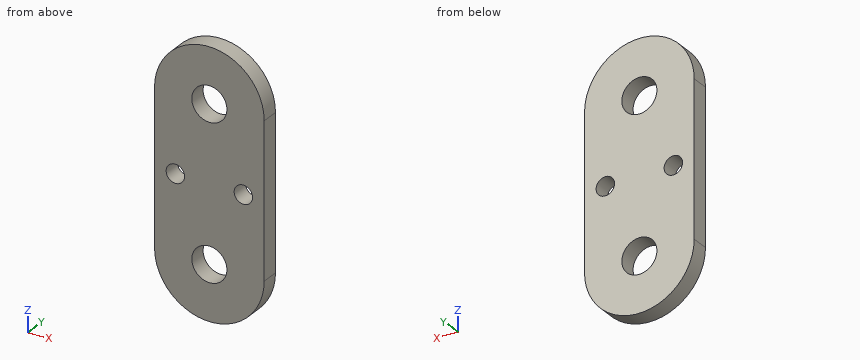
```python
from build123d import *

# Parameters (mm, degrees)
SKETCH1_R           = 12.5
SKETCH1_R_2         = 4
SKETCH1_R_3         = 2.1
BOSS_EXTRUDE1_DEPTH = 4


with BuildPart() as part:
    # Sketch1 → Boss-Extrude1 (new body)
    with BuildSketch(Plane(origin=(0, 0, 0), x_dir=(1, 0, 0), z_dir=(0, 1, 0))):
        with Locations((0, 17.5)):
            Circle(SKETCH1_R)
        with Locations((0, 17.5)):
            Circle(SKETCH1_R_2, mode=Mode.SUBTRACT)
        with BuildLine():
            ThreePointArc((-12.5, -17.5), (0, -5), (12.5, -17.5))
            Line((12.5, -17.5), (12.5, 17.5))
            ThreePointArc((12.5, 17.5), (-1.8e-08, 5), (-12.5, 17.500000037))
            Line((-12.5, 17.500000037), (-12.5, -17.5))
        make_face()
        with Locations((-7.75, 0)):
            Circle(SKETCH1_R_3, mode=Mode.SUBTRACT)
        with Locations((7.75, 0)):
            Circle(SKETCH1_R_3, mode=Mode.SUBTRACT)
        with Locations((0, -17.5)):
            Circle(SKETCH1_R)
        with Locations((0, -17.5)):
            Circle(SKETCH1_R_2, mode=Mode.SUBTRACT)
    extrude(amount=BOSS_EXTRUDE1_DEPTH)


solid = part.part
```
Could you check a few things on this model? Use its own coordinates, in mm. Coordinates: 2 decimals unless noted, no trailing zeros. Loops run counter-clockwise (first coordinate to the right, second up) from the corner with the lowest first, then second, coordinate; pieces in that order, holes last.
1) Please list where these lines run through material, in increasing order: line 1 along Z through (x, y) = (0, 3.2); line 2 along X through (y, z) = (1.5, 0); line 3 along X through (y, z) = (1.2, 17.5).
Reported:
line 1: z = -30 to -21.5, -13.5 to 13.5, 21.5 to 30
line 2: x = -12.5 to -9.85, -5.65 to 5.65, 9.85 to 12.5
line 3: x = -12.5 to -4, 4 to 12.5
2) Imagine slicing it at D-D (z = -19). List the corners of the cut face in (x, y) for me, and give its area (3 significant figures).
Reported:
outline: (-12.41, 0) - (-3.71, 0) - (-3.71, 4) - (-12.41, 4) - close; (3.71, 0) - (12.41, 0) - (12.41, 4) - (3.71, 4) - close
area: 69.6 mm2
3) Imagine slicing it at C-C (x = -7.75). List the corners of the cut face in (y, z) for me.
Reported:
outline: (0, -27.31) - (4, -27.31) - (4, -2.1) - (0, -2.1) - close; (0, 2.1) - (4, 2.1) - (4, 27.31) - (0, 27.31) - close
4) Imagine slicing it at A-A (y = 2.05). List the corners of the cut face in (x, z) for me.
Reported:
outline: (-12.5, -17.5) arc R12.5 ccw to (12.5, -17.5) - (12.5, 17.5) arc R12.5 ccw to (-12.5, 17.5) - close; hole circle Ø4.2 at (-7.75, 0); hole circle Ø8 at (0, -17.5); hole circle Ø8 at (0, 17.5); hole circle Ø4.2 at (7.75, 0)
5) Will these pins go through, and if not, where does the flat tip stop? pin 1 Ø2.5 at (x, z) = (7.75, 0) entering from -Y; pin 2 Ø1.5 at (y, z) = (3, -20) entering from +X; pin 3 Ø1 at (x, y) = (3, 3) entering from -Z.
Reported:
pin 1: passes through
pin 2: stops at x = 12.38
pin 3: stops at z = -29.75
6) Imagine slicing it at B-B (x = 0). List the corners of the cut face in (y, z) for me, and give its area (3 significant figures).
Reported:
outline: (0, -30) - (4, -30) - (4, -21.5) - (0, -21.5) - close; (0, -13.5) - (4, -13.5) - (4, 13.5) - (0, 13.5) - close; (0, 21.5) - (4, 21.5) - (4, 30) - (0, 30) - close
area: 176 mm2
